```python
from build123d import *

# Parameters (mm, degrees)
SKETCH_1_W          = 25
SKETCH_1_H          = 50
EXTRUDE_1_DEPTH     = 950
SKETCH_2_R          = 4
CUT_EXTRUDE_1_DEPTH = 50
CUT_EXTRUDE_START   = -50
SKETCH_3_R          = 4
CUT_EXTRUDE_2_DEPTH = 50


with BuildPart() as part:
    # Эскиз1 → Бобышка-Вытянуть1 (new body)
    with BuildSketch(Plane(origin=(0, 0, 0), x_dir=(1, 0, 0), z_dir=(0, 1, 0))):
        Rectangle(SKETCH_1_W, SKETCH_1_H)
    extrude(amount=EXTRUDE_1_DEPTH)

    # Эскиз2 → Вырез-Вытянуть1 (cut)
    with BuildSketch(Plane.XZ):
        with Locations(Location((0, 0, 0), (0, 0, 270))):
            Circle(SKETCH_2_R)
    extrude(amount=-CUT_EXTRUDE_1_DEPTH, mode=Mode.SUBTRACT)

    # Эскиз3 → Вырез-Вытянуть2 (cut)
    with BuildSketch(Plane(origin=(0, 950, 0), x_dir=(1, 0, 0), z_dir=(0, 1, 0)).offset(CUT_EXTRUDE_START)):
        with Locations(Location((0, 0, 0), (0, 0, 90))):
            Circle(SKETCH_3_R)
    extrude(amount=CUT_EXTRUDE_2_DEPTH, mode=Mode.SUBTRACT)


solid = part.part
```
Verification items for the finished model (mm, model axes). Coordinates: 2 decimals unless noted, no trailing zeros. Loops run counter-clockwise (first coordinate to the right, second up) from the corner with the lowest first, then second, coordinate; pieces in that order, holes last. Notation, with made-up numbers: (41, -36) -> (47, -36) arc R9 ccw to (47, -26) -> close; hole circle Ø2 at (81.25, 74.25). An arc over 180 degrees is marked (long way). Answer in a Markdown table with one row per item. Add a question column.
1. Depth check by flat-ended pin: P1, Ø7, axis at x = 0, z = 0, coming from the +Y side. Enter the tip coordinate at first touch or a pass-through.
2. Material ranges on probe 1 along X at (y, z) = (39.5, 0); probe 2 along Y at (x, z) = (-1.5, -3.5), recorded low to high. Write a range as [from, to].
3. Section check A-A, the plane x = 0. Enter the section's corners in (y, z), then the cut area to 3 significant figures.
Derived:
| question | item | result |
|---|---|---|
| 1 | P1 | stops at y = 900 |
| 2 | probe 1 | x = [-12.5, -4], [4, 12.5] |
| 2 | probe 2 | y = [50, 900] |
| 3 | outline | (0, -25) -> (950, -25) -> (950, -4) -> (900, -4) -> (900, 4) -> (950, 4) -> (950, 25) -> (0, 25) -> (0, 4) -> (50, 4) -> (50, -4) -> (0, -4) -> close |
| 3 | area | 46,700 mm² |
